Read the model definition and answer for the solid it produces. Units are mm, in the model's axes. A direction names the side the tool comes from. Coordinates: 2 decimals unless noted, no trailing zeros. Write each loop counter-clockwise with the first axis right and the second up, starting at its lowest first coordinate (ties: lowest second). Pieces come first, ordered by that corner, then holes. Notation, with made-up numbers: (2.5, -32.75) - (39.5, -32.75) arc R28 ccw to (39.5, -13.75) - close; hole circle Ø10 at (70.25, 70.5). An arc over 180 degrees is marked (long way). Return JSON: item names as keys, results as strings.
```python
from build123d import *

# Parameters (mm, degrees)
BOSS_EXTRUDE1_DEPTH = 2.5
FILLET1_R           = 5
SKETCH3_R           = 1.6
SKETCH3_R_2         = 2
CUT_EXTRUDE1_DEPTH  = 6
SKETCH3_4_R         = 1.6
CUT_EXTRUDE2_DEPTH  = 10
SKETCH4_R           = 2.5
CUT_EXTRUDE3_DEPTH  = 2


with BuildPart() as part:
    # Sketch2 → Boss-Extrude1 (new body, symmetric)
    with BuildSketch(Plane.XY):
        with BuildLine():
            ThreePointArc((17, 0), (12.02081528, 12.02081528), (0, 17))
            Line((0, 17), (0, 5.5))
            ThreePointArc((0, 5.5), (3.889087297, 3.889087297), (5.5, 0))
            ThreePointArc((5.5, 0), (3.889087297, -3.889087297), (0, -5.5))
            Line((0, -5.5), (0, -17))
            ThreePointArc((0, -17), (12.02081528, -12.02081528), (17, 0))
        make_face()
        with BuildLine():
            Line((148, 17), (0, 17))
            ThreePointArc((0, 17), (12.02081528, 12.02081528), (17, 0))
            ThreePointArc((17, 0), (12.02081528, -12.02081528), (0, -17))
            Line((0, -17), (148, -17))
            Line((148, -17), (148, 17))
        make_face()
        with BuildLine():
            Line((0, 5.5), (0, 17))
            ThreePointArc((0, 17), (-12.02081528, 12.02081528), (-17, 0))
            Line((-17, 0), (-5.5, 0))
            ThreePointArc((-5.5, 0), (-3.889087297, 3.889087297), (0, 5.5))
        make_face()
        with BuildLine():
            Line((-5.5, 0), (-17, 0))
            ThreePointArc((-17, 0), (-12.02081528, -12.02081528), (0, -17))
            Line((0, -17), (0, -5.5))
            ThreePointArc((0, -5.5), (-3.889087297, -3.889087297), (-5.5, 0))
        make_face()
        with BuildLine():
            Line((0, 5.5), (0, 17))
            ThreePointArc((0, 17), (-12.02081528, 12.02081528), (-17, 0))
            Line((-17, 0), (-5.5, 0))
            ThreePointArc((-5.5, 0), (-3.889087297, 3.889087297), (0, 5.5))
        make_face()
        with BuildLine():
            Line((-5.5, 0), (-17, 0))
            ThreePointArc((-17, 0), (-12.02081528, -12.02081528), (0, -17))
            Line((0, -17), (0, -5.5))
            ThreePointArc((0, -5.5), (-3.889087297, -3.889087297), (-5.5, 0))
        make_face()
    extrude(amount=BOSS_EXTRUDE1_DEPTH, both=True)

    # Fillet1
    fillet1_edges = [part.edges().sort_by_distance(p)[0] for p in [
        (148, 17, -1.25),
        (148, -17, -1.25),
    ]]
    fillet(fillet1_edges, radius=FILLET1_R)

    # Sketch3 → Cut-Extrude1 (cut, through all)
    with BuildSketch(Plane(origin=(0, 0, -2.5), x_dir=(-1, 0, 0), z_dir=(0, 0, -1))):
        with BuildLine():
            Line((-97.609487516, 17), (-98.390512484, 17))
            ThreePointArc((-98.390512484, 17), (-99.537449186, 15.303149803), (-98, 13.95))
            ThreePointArc((-98, 13.95), (-96.462550814, 15.303149803), (-97.609487516, 17))
        make_face()
        with BuildLine():
            ThreePointArc((-141.390512484, 17), (-141, 13.95), (-140.609487516, 17))
            Line((-140.609487516, 17), (-141.390512484, 17))
        make_face()
        with Locations((-87.5, 15)):
            Circle(SKETCH3_R)
        with Locations((-65, 12)):
            Circle(SKETCH3_R_2)
        with BuildLine():
            Line((-141.390512484, -17), (-140.609487516, -17))
            ThreePointArc((-140.609487516, -17), (-141, -13.95), (-141.390512484, -17))
        make_face()
        with BuildLine():
            ThreePointArc((-97.609487516, -17), (-98, -13.95), (-98.390512484, -17))
            Line((-98.390512484, -17), (-97.609487516, -17))
        make_face()
        with BuildLine():
            Line((-10.574175964, 14.5), (-15.574175964, 14.5))
            ThreePointArc((-15.574175964, 14.5), (-17.074175964, 13), (-15.574175964, 11.5))
            Line((-15.574175964, 11.5), (-10.574175964, 11.5))
            ThreePointArc((-10.574175964, 11.5), (-9.074175964, 13), (-10.574175964, 14.5))
        make_face()
        with Locations((-87.5, -15)):
            Circle(SKETCH3_R)
        with Locations((-65, -12)):
            Circle(SKETCH3_R_2)
    extrude(amount=-CUT_EXTRUDE1_DEPTH, mode=Mode.SUBTRACT)

    # Sketch3_4 → Cut-Extrude2 (cut)
    with BuildSketch(Plane(origin=(0, 0, -2.5), x_dir=(-1, 0, 0), z_dir=(0, 0, -1))):
        with Locations((-42.5, -15)):
            Circle(SKETCH3_4_R)
        with Locations((-42.5, 15)):
            Circle(SKETCH3_4_R)
    extrude(amount=-CUT_EXTRUDE2_DEPTH, mode=Mode.SUBTRACT)

    # Sketch4 → Cut-Extrude3 (cut)
    with BuildSketch(Plane(origin=(0, 0, -2.5), x_dir=(-1, 0, 0), z_dir=(0, 0, -1))):
        with Locations((-42.5, 15)):
            Circle(SKETCH4_R)
        with Locations((-42.5, -15)):
            Circle(SKETCH4_R)
    extrude(amount=-CUT_EXTRUDE3_DEPTH, mode=Mode.SUBTRACT)


solid = part.part
```
(1) A cutting plane is placed at C-C (y = -2.5). Determine the outline of the cut face in (x, z), and give its area (3 significant figures).
Answer:
{"outline": "(-16.82, -2.5) - (-4.9, -2.5) - (-4.9, 2.5) - (-16.82, 2.5) - close; (4.9, -2.5) - (148, -2.5) - (148, 2.5) - (4.9, 2.5) - close", "area": "775 mm²"}
(2) A cutting plane is placed at A-A (x = -2). Determine the outline of the cut face in (y, z).
Answer:
{"outline": "(-16.88, -2.5) - (-5.12, -2.5) - (-5.12, 2.5) - (-16.88, 2.5) - close; (5.12, -2.5) - (16.88, -2.5) - (16.88, 2.5) - (5.12, 2.5) - close"}
(3) Determine the mould class of faces 1 (the face through (148, 0, 0)), 2 (the face through (66.474, -10.648, -0.035)), 3 (the face through (119, -17, 0)) for opening direction Y: +Y half, -Y half, draft (parallel to the pull), parting line (faces both ways), or undercut.
Answer:
{"face 1": "draft", "face 2": "undercut", "face 3": "-Y half"}
(4) Which of the six approach directions +Z, -Z, +X, -X, +Y, -Y give full straight-line access (tool end or side, diameter ignored) to faces 4 (the face through (17.074, 13.033, -0.035)), 5 (the face through (48, -17, 0)), 6 (the face through (41, -14, -0.5))?
Answer:
{"face 4": "+Z, -Z", "face 5": "+Z, -Z, +X, -X, -Y", "face 6": "-Z"}
(5) Flat-ended cylindrical pins translate along their axes: P1, Ø5, axis at x = 43, y = -14, coming from the -Z side; P2, Ø2.5, axis at x = 65, y = -12, coming from the +Z side; P3, Ø3, axis at y = -10, z = 1, coming from the -X side. Find the tip coordinate at first contact, or state that the pin passes through.
Answer:
{"P1": "z = -2.5", "P2": "through", "P3": "x = -14.72"}
(6) A cutting plane is placed at B-B (z = 1.7). State how many separate pieces and enclosed holes the cut face has, and give its area (3 significant figures).
Answer:
{"separate pieces": "1", "enclosed holes": "8", "area": "5,270 mm²"}
(7) Straight lines are drawn through the part: line 1 (Y direction, x = 65, z = 0); line 2 (Y direction, x = 87.5, z = -1.05); line 3 (X direction, y = -13, z = -1.85). For each, find the intervals that lie inside material, in ascending order. Write a range as from..to.
Answer:
{"line 1": "-17..-14, -10..10, 14..17", "line 2": "-17..-16.6, -13.4..13.4, 16.6..17", "line 3": "-10.95..41, 44..63.27, 66.73..147.9"}
